Design review of the part built by this model. Coordinates are the model's own, in mm. A direction names the side the tool comes from. Coordinates: 2 decimals unless noted, no trailing zeros. Write each loop counter-clockwise with the first axis right and the second up, starting at its lowest first coordinate (ties: lowest second). Pieces come first, ordered by that corner, then holes. Notation, with made-up numbers: M 11.25,11.25 L 51.25,11.25 A22 cw 51.25,41.25 Z; hole C 70.5,-5 d3. An arc over 180 degrees is marked long. One line per question, with ' | ' between items.
from build123d import *

# Parameters (mm, degrees)
F0_W      = 139.9
F0_H      = 75
F1_DEPTH  = 5
F2_W      = 139.9
F2_H      = 5
F5_DEPTH  = 65.5
F3_W      = 4.8456325173
F3_H      = 70
F6_DEPTH  = 65.5
F4_W      = 4.7526705265
F4_H      = 69.843
F7_DEPTH  = 65.5
F9_W      = 5
F9_H      = 65.0515219681
F10_DEPTH = 132.6
F11_R     = 8.3357715152
F12_DEPTH = 7.5


with BuildPart() as f1:
    # F0 (on Top) → F1 (new body)
    with BuildSketch(Plane.XY):
        with Locations((4.7975996614, -37.6802921295)):
            Rectangle(F0_W, F0_H)
    extrude(amount=F1_DEPTH)

    # F2 (on face) → F5 (join)
    with BuildSketch(Plane.XY.offset(5)):
        with Locations((4.7975996614, -2.6802921295)):
            Rectangle(F2_W, F2_H)
    extrude(amount=F5_DEPTH)

    # F3 (on face) → F6 (join)
    with BuildSketch(Plane.XY.offset(5)):
        with Locations((-62.72958408, -40.1802921295)):
            Rectangle(F3_W, F3_H)
    extrude(amount=F6_DEPTH)

    # F4 (on face) → F7 (join)
    with BuildSketch(Plane.XY.offset(5)):
        with Locations((72.3712643981, -40.1582837973)):
            Rectangle(F4_W, F4_H)
    extrude(amount=F7_DEPTH)

    # F9 (on face) → F10 (join)
    with BuildSketch(Plane.YZ.offset(-60.3067678213)):
        with Locations((-72.3428228498, 37.525760984)):
            Rectangle(F9_W, F9_H)
    extrude(amount=F10_DEPTH)

    # F11 (on face) → F12 (join)
    with BuildSketch(Plane.XZ.offset(74.8428228498)):
        with Locations((0, 40.6753867865)):
            Circle(F11_R)
    extrude(amount=F12_DEPTH)


solid = f1.part
1. Take a section at D-D (x = 65). Write out the cut boundary in (y, z).
Answer sheet:
outline: M -75.18,0 L -0.18,0 L -0.18,70.5 L -5.18,70.5 L -5.18,5 L -69.84,5 L -69.84,70.05 L -74.84,70.05 L -74.84,5 L -75.18,5 Z
2. Take a section at C-C (z = 62). Write out the cut boundary in (x, y).
Answer sheet:
outline: M -65.15,-75.18 L -60.31,-75.18 L -60.31,-74.84 L 69.99,-74.84 L 69.99,-75.08 L 74.75,-75.08 L 74.75,-5.24 L 69.99,-5.24 L 69.99,-69.84 L -60.31,-69.84 L -60.31,-5.18 L 74.75,-5.18 L 74.75,-0.18 L -65.15,-0.18 Z
3. Insertion check: pin 1 Ø1 at (x, z) = (-46, 60) entering from -Y; pin 2 Ø1 at (x, y) = (2.5, -10.5) entering from +Z; pin 3 Ø12 at (x, y) = (-26, -23.5) entering from -Z; pin 4 Ø4 at (x, y) = (30, -73.5) entering from +Z. Each pin has a flat end and moves straight along its axis. Give the tip position at first contact, or say it passes through.
Answer sheet:
pin 1: y = -74.84 | pin 2: z = 5 | pin 3: z = 0 | pin 4: z = 70.05
4. Take a section at B-B (x = 0). Write out the cut boundary in (y, z), then the cut area to 3 significant figures.
Answer sheet:
outline: M -82.34,32.34 L -74.84,32.34 L -74.84,5 L -75.18,5 L -75.18,0 L -0.18,0 L -0.18,70.5 L -5.18,70.5 L -5.18,5 L -69.84,5 L -69.84,70.05 L -74.84,70.05 L -74.84,49.01 L -82.34,49.01 Z | area: 1,150 mm^2
5. Draft analysis for pull direction X (two halves, no side actions). For faces 4 (the face through (-65.152, -38, 35)), 5 (the face through (4, -74.843, 30)), 6 (the face through (4, -37, 0)), state which applies: pulls with the +X half, pulls with the -X half, needs draft (parallel to the pull), parting line crosses it, or undercut.
Answer sheet:
face 4: pulls with the -X half | face 5: undercut | face 6: needs draft
6. Tool access review of faces 1 (the face through (4, -72, 70.052)), 2 (the face through (69.995, -41, 37)), 3 (the face through (-1.81, -78.54, 32.54)): name each direction out of +Z, -Z, +X, -X, +Y, -Y from which nothing blocks a thin tool from reaching the whole face with its end or side.
Answer sheet:
face 1: +Z, -Y | face 2: +Z | face 3: -Y
7. Take a section at A-A (y = -39). Write out the cut boundary in (x, z), then the cut area to 3 significant figures.
Answer sheet:
outline: M -65.15,0 L 74.75,0 L 74.75,70.5 L 69.99,70.5 L 69.99,5 L -60.31,5 L -60.31,70.5 L -65.15,70.5 Z | area: 1,330 mm^2
8. To check wall thickness, follow line 1 along X through (y, z) = (-13, 59); line 2 along Y through (x, z) = (49, 10.5); line 3 along Y through (x, z) = (-0.5, 46). State the ranges of each line that lie inside material, in increasing order. Write a range as [from, to].
Answer sheet:
line 1: [-65.15, -60.31], [69.99, 74.75] | line 2: [-74.84, -69.84], [-5.18, -0.18] | line 3: [-82.34, -69.84], [-5.18, -0.18]
